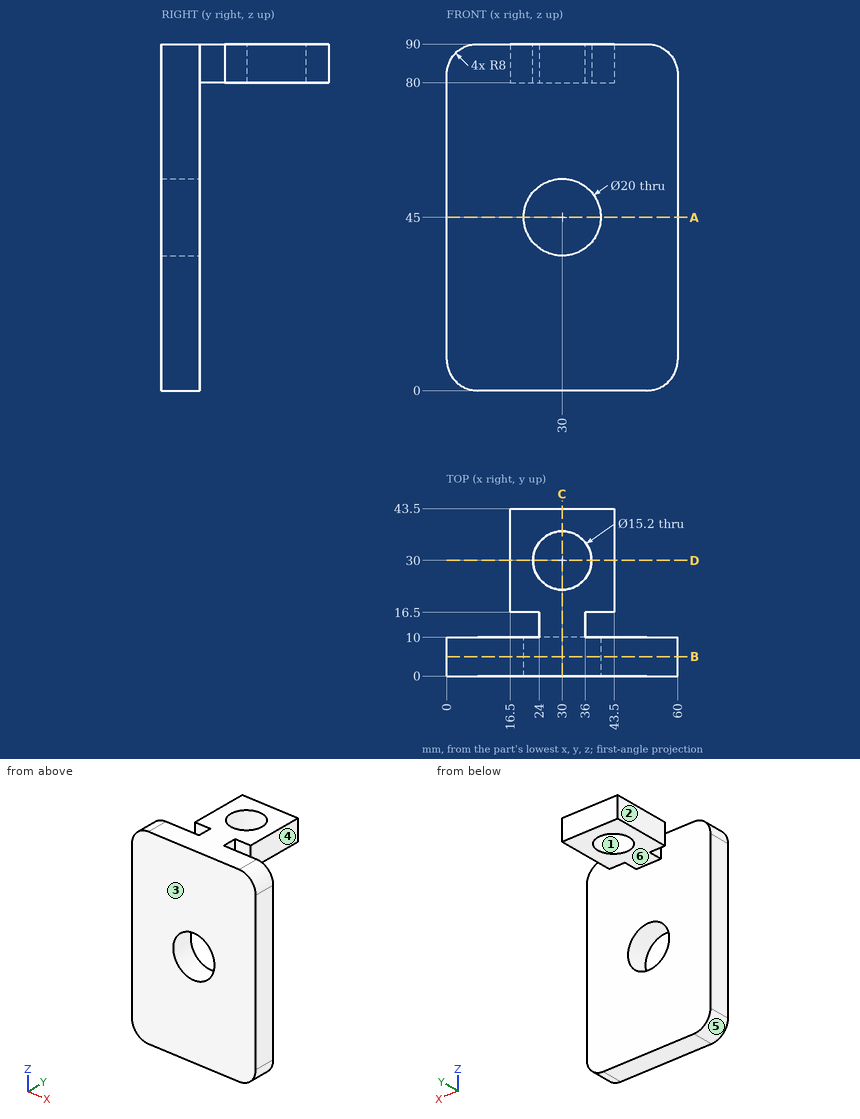
The drawing under review shows one solid part. Ordinate dimensions are in mm from its lowest x, y, z. A direction names the side the tool comes from. Coordinates: 2 decimals unless noted, no trailing zeros. Loops run counter-clockwise (first coordinate to the right, second up) from the corner with the lowest first, then second, coordinate; pieces in that order, holes last.
Item 1: Add section B-B (y = 5). Write out the cut boundary in (x, z).
Completed:
outline: (0, 8) arc R8 ccw to (8, 0) - (52, 0) arc R8 ccw to (60, 8) - (60, 82) arc R8 ccw to (52, 90) - (8, 90) arc R8 ccw to (0, 82) - close; hole circle Ø20 at (30, 45)
Item 2: Add section D-D (y = 30). Write out the cut boundary in (x, z), and give its area (3 significant figures).
Completed:
outline: (16.5, 80) - (22.4, 80) - (22.4, 90) - (16.5, 90) - close; (37.6, 80) - (43.5, 80) - (43.5, 90) - (37.6, 90) - close
area: 118 mm2
Item 3: For the marked faces 4, 5 and 6, list the 3-axis set-ups (+Z, -Z, +X, -X, +Y, -Y) from which the entire face can be reached by the end or side of a thin tool; tool diameter is ignored.
Completed:
face 4: +Z, -Z, +X, +Y
face 5: -Z, -X, +Y, -Y
face 6: -Z, +X, -X, +Y
Item 4: Wall thickness on L1, parallel to X at y = 4, z = 45; L2, parallel to Z at x = 30, y = 5.25; L3, parallel to X at y = 30, z = 86: over which ranges is each line inside the solid? List them lowest first.
Completed:
L1: x = 0 to 20, 40 to 60
L2: z = 0 to 35, 55 to 90
L3: x = 16.5 to 22.4, 37.6 to 43.5
Item 5: Clearance check with flat-ended pins moving along their axes: pin 1 (18 mm diameter, centred on x = 18, z = 64, fed in from +Y); pin 2 (8 mm diameter, centred on x = 27, y = 33.5, fed in from -Z); pin 3 (9 mm diameter, centred on x = 30, y = 30, fed in from +Z); pin 4 (3 mm diameter, centred on y = 14, z = 84, fed in from -X). State where each tip first meets the part, or that it passes through.
Completed:
pin 1: stops at y = 10
pin 2: stops at z = 80
pin 3: passes through
pin 4: stops at x = 24
Item 6: Add section A-A (z = 45). Write out the cut boundary in (x, y).
Completed:
outline: (0, 0) - (20, 0) - (20, 10) - (0, 10) - close; (40, 0) - (60, 0) - (60, 10) - (40, 10) - close
Item 7: Draft analysis for pull direction Y (two halves, no side actions). For the marked faces 1, 2 and 3, state which applies: pulls with the +Y half, pulls with the -Y half, needs draft (parallel to the pull), parting line crosses it, or undercut.
Completed:
face 1: undercut
face 2: needs draft
face 3: pulls with the -Y half
Item 8: Add section C-C (x = 30). Write out the cut boundary in (y, z).
Completed:
outline: (0, 0) - (10, 0) - (10, 35) - (0, 35) - close; (0, 55) - (10, 55) - (10, 80) - (22.4, 80) - (22.4, 90) - (0, 90) - close; (37.6, 80) - (43.5, 80) - (43.5, 90) - (37.6, 90) - close
